Part model, mm, in its own coordinate system. A direction names the side the tool comes from. Give positions to 0.01 mm unless a question says otherwise; leave off trailing zeros. Order: outer loops, then holes, each group sorted by start corner. A loop starts at its lowest first (then second) coordinate and runs counter-clockwise, first axis right, second up. Notation, with made-up numbers: M 89.5,38 L 104.5,38 A23 cw 104.5,61 Z; hole C 39,31 d6. An arc over 180 degrees is marked long. Return JSON: item names as keys, results as strings.
Autodesk Inventor part; units mm, degrees
ref_plane "YZ Plane" through (0, 0, 0) normal (1, 0, 0) x (0, 1, 0)
ref_plane "XZ Plane" through (0, 0, 0) normal (0, 1, 0) x (-1, 0, 0)
ref_plane "XY Plane" through (0, 0, 0) normal (0, 0, 1) x (1, 0, 0)
sketch "Sketch1" plane through (0, 0, 0) normal (0, 1, 0) x (-1, 0, 0)
  line L0 (-200, 325) -> (200, 325)
  line L1 (200, 325) -> (200, -325)
  line L2 (200, -325) -> (-200, -325)
  line L3 (-200, -325) -> (-200, 325)
  line L4 (-200, 325) -> (200, -325) construction
  line L5 (200, 325) -> (-200, -325) construction
  point P0 (0, 0)
  dimension "d0" = 650
  dimension "d1" = 400
extrude "Extrusion1" add sketch "Sketch1" along normal blind 5
sketch "Sketch2" plane through (200, 0, -325) normal (0, 0, -1) x (-1, 0, 0)
  line L0 (0, 5) -> (400, 5)
  line L1 (400, 5) -> (395, 5)
  line L2 (395, 5) -> (395, 505)
  line L3 (395, 505) -> (400, 505)
  line L4 (400, 505) -> (400, 5)
  point P0 (200, 0)
  dimension "d4" = 5
  dimension "d5" = 500
extrude "Extrusion2" add sketch "Sketch2" against normal blind 400
sketch "Sketch3" plane through (-195, 5, -325) normal (1, 0, 0) x (0, 0, -1)
  line L0 (-400, 0) -> (-400, 500)
  line L1 (0, 500) -> (0, 0)
  point P0 (-325, -5)
  point P1 (-385, 463.2751)
  point P2 (-15, 463.2751)
  point P3 (-15, 293.2751)
  point P4 (-385, 293.2751)
  dimension "d8" = 15
  dimension "d9" = 15
  dimension "d10" = 170
hole "Hole1" at (-195, 468.2751, 60) at (-195, 468.2751, -310) at (-195, 298.2751, -310) at (-195, 298.2751, 60) direction (-1, 0, 0) diameter 10 end through all
properties part number "df"
Q1. Band-saw the part on B-B (y = 40.5). Give the cut face in (x, z), then the cut area to 3 significant figures.
Established:
{"outline": "M -200,-325 L -195,-325 L -195,75 L -200,75 Z", "area": "2,000 mm²"}
Q2. Band-saw the part on A-A (z = -167.5). Give the cut face in (x, y).
Established:
{"outline": "M -200,0 L 200,0 L 200,5 L -195,5 L -195,505 L -200,505 Z"}
Q3. 3-axis set-ups, long thin cutter, end or side, ignore diameter. For faces 1 (the flat face through (3, 0, 5)), 2 (the flat face through (-195, 252, -128)): which of +Z, -Z, +X, -X, +Y, -Y reach the whole face in a straight line?
Established:
{"face 1": "+Z, -Z, +X, -X, -Y", "face 2": "+Z, -Z, +X, +Y"}
Q4. Pin check, flat tips, straight feed: pin 1 (3 mm diameter, centred on x = 81.5, z = 28, fed in from +Y); pin 2 (11.5 mm diameter, centred on y = 298.28, z = -310, fed in from +X); pin 3 (2.5 mm diameter, centred on x = -197, y = 133.5, fed in from +Z). Stop position of each tip, or through.
Established:
{"pin 1": "stops at y = 5", "pin 2": "stops at x = -195", "pin 3": "stops at z = 75"}
Q5. Band-saw the part on C-C (x = 30.5). Give the cut face in (y, z), then the cut area to 3 significant figures.
Established:
{"outline": "M 0,-325 L 5,-325 L 5,325 L 0,325 Z", "area": "3,250 mm²"}
Q6. Probe line 1 along Y through (x, z) = (-196, 60); line 2 along Y through (x, z) = (1, 237); line 3 along X through (y, z) = (104, 12). List the from-to ranges inside material, lowest first.
Established:
{"line 1": "y = 0 to 293.28, 303.28 to 463.28, 473.28 to 505", "line 2": "y = 0 to 5", "line 3": "x = -200 to -195"}
